```python
from build123d import *

# Parameters (mm, degrees)
F0_R     = 254
F1_DEPTH = 254


with BuildPart() as f1:
    # F0 (on Front) → F1 (new body)
    with BuildSketch(Plane.XZ):
        with BuildLine():
            Line((0, 381), (0, 127))
            ThreePointArc((0, 127), (37.197439, 37.197439), (127, 0))
            Line((127, 0), (1778, 0))
            Line((1778, 0), (1778, 381))
            Line((1778, 381), (2047.407684, 650.407684))
            Line((2047.407684, 650.407684), (1819.527595, 878.287772))
            Line((1819.527595, 878.287772), (1550.119911, 608.880089))
            Line((1550.119911, 608.880089), (1370.514789, 788.485211))
            Line((1370.514789, 788.485211), (1639.922472, 1057.892895))
            Line((1639.922472, 1057.892895), (1412.407684, 1285.407684))
            Line((1412.407684, 1285.407684), (1143, 1016))
            Line((1143, 1016), (889, 1016))
            Line((889, 1016), (889, 762))
            Line((889, 762), (762, 762))
            Line((762, 762), (762, 1016))
            Line((762, 1016), (381, 1016))
            ThreePointArc((381, 1016), (291.197439, 978.802561), (254, 889))
            Line((254, 889), (254, 508))
            Line((254, 508), (127, 508))
            ThreePointArc((127, 508), (37.197439, 470.802561), (0, 381))
        make_face()
        with Locations((825.5, 381)):
            Circle(F0_R, mode=Mode.SUBTRACT)
    extrude(amount=F1_DEPTH)


solid = f1.part
```
Part model, mm, in its own coordinate system. A direction names the side the tool comes from. Round coordinates to 2 decimals unless told otherwise and drop trailing zeros. Loops run counter-clockwise (first coordinate to the right, second up) from the corner with the lowest first, then second, coordinate; pieces in that order, holes last. Notation, with made-up numbers: (49, 81) -> (71, 81) arc R36 cw to (71, 117) -> close; hole circle Ø4 at (26, 42). An arc over 180 degrees is marked (long way). Use CSV: the item, a comma, the result in double quotes. Start each with the question number.
1) Cut at A-A, the plane x = 825.5. Write the cut outline in (y, z).
2) Cut at C-C, the plane y = -49. Write the cut outline in (x, z).
3) Pull direction Z, two halves, no side cores. Call faces 6 (the flat face through (1935.063, -125.222, 762.753)), 7 (the flat face through (889, -125, 891)), 8 (the flat face through (1503.33, -125.22, 921.3)), 9 (the cylindrical face through (36.215, -125.222, 38.19)): +Z half, -Z half, draft (parallel to the pull), parting line (faces both ways), or undercut.
4) Which spindle directions (+Z, -Z, +X, -X, +Y, -Y) get a long thin tool onto all of the face, cutting with end or side? Do faces 1 (the flat face through (1527.758, -125.222, 1170.058)), 2 (the flat face through (762, -125, 887)), 3 (the flat face through (1018, -125, 1016)), 4 (the flat face through (1462, -125, 697)), 5 (the flat face through (1778, -125, 188)). Say none if no direction does.
5) Drop flat-ended pins along their axis: P1, Ø4, axis at y = -65, z = 146, coming from the +X side; P2, Ø5, axis at y = -206, z = 1122.5, coming from the +X side; P3, Ø8, axis at x = 1720.5, y = -105.5, coming from the +Z side. Give the stop position or say it passes through.
6) Cut at D-D, the plane z = 815.5. Write the cut outline in (x, y), plus the area to 3 significant figures.
7) Cut at B-B, the plane z = 227. Write the cut outline in (x, y).
8) Wall check: L1, parallel to Z at x = 825, y = -81; L2, parallel to Z at x = 546, y = -31; L3, parallel to Z at x = 1528, y = -64.5. Give the ranges that are in metal, low to high. Write a range as [from, to].
Determined:
1,outline,"(-254, 0) -> (0, 0) -> (0, 127) -> (-254, 127) -> close; (-254, 635) -> (0, 635) -> (0, 762) -> (-254, 762) -> close"
2,outline,"(0, 127) arc R127 ccw to (127, 0) -> (1778, 0) -> (1778, 381) -> (2047.41, 650.41) -> (1819.53, 878.29) -> (1550.12, 608.88) -> (1370.51, 788.49) -> (1639.92, 1057.89) -> (1412.41, 1285.41) -> (1143, 1016) -> (889, 1016) -> (889, 762) -> (762, 762) -> (762, 1016) -> (381, 1016) arc R127 ccw to (254, 889) -> (254, 508) -> (127, 508) arc R127 ccw to (0, 381) -> close; hole circle Ø508 at (825.5, 381)"
3,face 6,"+Z half"
3,face 7,"draft"
3,face 8,"undercut"
3,face 9,"-Z half"
4,face 1,"+Z, +X, +Y, -Y"
4,face 2,"+Z, +Y, -Y"
4,face 3,"+Z, -X, +Y, -Y"
4,face 4,"+Y, -Y"
4,face 5,"-Z, +X, +Y, -Y"
5,P1,"stops at x = 1778"
5,P2,"stops at x = 1577.82"
5,P3,"stops at z = 783.26"
6,outline,"(254, -254) -> (762, -254) -> (762, 0) -> (254, 0) -> close; (889, -254) -> (1397.53, -254) -> (1397.53, 0) -> (889, 0) -> close; (1756.74, -254) -> (1882.32, -254) -> (1882.32, 0) -> (1756.74, 0) -> close"
6,area,"290,000 mm2"
7,outline,"(0, -254) -> (623.51, -254) -> (623.51, 0) -> (0, 0) -> close; (1027.49, -254) -> (1778, -254) -> (1778, 0) -> (1027.49, 0) -> close"
8,L1,"z = [0, 127], [635, 762]"
8,L2,"z = [0, 1016]"
8,L3,"z = [0, 631], [945.97, 1169.82]"
